Autodesk Inventor part; units mm, degrees
ref_plane "작업 평면1" through (80, 0, 4.95) normal (0, 0, 1) x (1, 0, 0)
ref_plane "YZ Plane" through (0, 0, 0) normal (1, 0, 0) x (0, 1, 0)
ref_plane "XZ Plane" through (0, 0, 0) normal (0, 1, 0) x (-1, 0, 0)
sketch "스케치1" plane through (0, 0, 0) normal (1, 0, 0) x (0, 1, 0)
  circle A0 centre (0, 0) radius 6
  dimension "d0" = 12
extrude "돌출1" add sketch "스케치1" along normal blind 80
sketch "스케치8" plane through (0, 0, 0) normal (-1, 0, 0) x (0, 0, 1)
  circle A0 centre (0, 0) radius 6
  circle A1 centre (0, 0) radius 4.95
  dimension "d26" = 9.9
extrude "돌출8" cut sketch "스케치8" against normal blind 18.6
sketch "스케치9" plane through (0, 0, 0) normal (-1, 0, 0) x (0, 0, 1)
  circle A0 centre (0, 0) radius 4.8
  circle A1 centre (0, 0) radius 4.95
  dimension "d29" = 9.6
extrude "돌출9" cut sketch "스케치9" against normal blind 9
sketch "스케치10" plane through (0, 0, 0) normal (-1, 0, 0) x (0, 0, 1)
  circle A0 centre (0, 0) radius 4.95
  circle A1 centre (0, 0) radius 4.8
  dimension "d32" = 9.9
extrude "돌출10" add sketch "스케치10" against normal blind 8
sketch "스케치11" plane through (80, 0, 0) normal (1, 0, 0) x (0, 0, -1)
  circle A0 centre (0, 0) radius 6
  circle A1 centre (0, 0) radius 4.95
  dimension "d35" = 9.9
extrude "돌출11" cut sketch "스케치11" against normal blind 26
sketch "스케치12" plane through (80, 0, 0) normal (1, 0, 0) x (0, 0, -1)
  circle A0 centre (0, 0) radius 4.95
  circle A1 centre (0, 0) radius 4.8
  dimension "d38" = 9.6
extrude "돌출12" cut sketch "스케치12" against normal blind 16.4
sketch "스케치13" plane through (80, 0, 0) normal (1, 0, 0) x (0, 0, -1)
  circle A0 centre (0, 0) radius 4.95
  circle A1 centre (0, 0) radius 4.8
  dimension "d41" = 9.9
extrude "돌출13" add sketch "스케치13" against normal blind 15.4
ref_plane "작업 평면1" through (80, 0, 4.95) normal (0, 0, 1) x (1, 0, 0)
sketch "스케치14" plane through (80, 0, 4.95) normal (0, 0, 1) x (1, 0, 0)
  line L0 (-1.3, -1.55) -> (-13.4, -1.55)
  line L1 (-13.4, -1.55) -> (-13.4, 1.55)
  line L2 (-13.4, 1.55) -> (-1.3, 1.55)
  line L3 (-1.3, 1.55) -> (-1.3, -1.55)
  line L4 (-15.4, 4.95) -> (-15.4, -4.95)
  line L5 (0, 4.95) -> (0, -4.95)
  line L6 (0, 0) -> (-15.4, 0)
  line L7 (-15.4, 4.8) -> (-15.4, -4.8)
  point P0 (-80, 0)
  dimension "d44" = 12.1
  dimension "d45" = 3.1
  dimension "d46" = 12.1
  dimension "d47" = 2
  dimension "d48" = 1.55
extrude "돌출14" cut sketch "스케치14" against normal blind 1.3
sketch "스케치15" plane through (54, 0, 0) normal (1, 0, 0) x (0, 0, -1)
  circle A0 centre (0, 0) radius 4.95
  circle A1 centre (0, 0) radius 6
  circle A2 centre (0, 0) radius 4.95
  circle A3 centre (0, 0) radius 4.95
  circle A4 centre (0, 0) radius 4.8
  dimension "d51" = 9.6
extrude "돌출15" cut sketch "스케치15" against normal blind 1 contours A0 | A1
sketch "스케치16" plane through (18.6, 0, 0) normal (-1, 0, 0) x (0, 0, 1)
  circle A0 centre (0, 0) radius 4.95
  circle A1 centre (0, 0) radius 6
  circle A2 centre (0, 0) radius 4.95
  circle A3 centre (0, 0) radius 4.8
  dimension "d54" = 9.6
extrude "돌출16" cut sketch "스케치16" against normal blind 1.1 contours A0 | A1
sketch "스케치17" plane through (19.7, 0, 0) normal (-1, 0, 0) x (0, 0, 1)
  circle A0 centre (0, 0) radius 4.8
  circle A1 centre (0, 0) radius 6
  circle A2 centre (0, 0) radius 4.95
  circle A3 centre (0, 0) radius 4.95
extrude "돌출17" cut sketch "스케치17" against normal blind 33.35 contours A1
properties part number "10PI축" material "철, 주조"
Model file for the job. Use its own axes, mm. A direction names the side the tool comes from. Give positions to 0.01 mm unless a question says otherwise; leave off trailing zeros. Write each loop counter-clockwise with the first axis right and the second up, starting at its lowest first coordinate (ties: lowest second). Pieces come first, ordered by that corner, then holes. Notation, with made-up numbers: M -15.75,-11 L -3.75,-11 A13 cw -3.75,8 Z; hole C 88.25,-1 d4. An arc over 180 degrees is marked long. One line per item, written item: value. Start each with the question number.
Q1. Drop flat-ended pins along their axis: pin 1 Ø0.8 at (x, z) = (71.5, 4.5) entering from +Y; pin 2 Ø3 at (x, y) = (46, 2) entering from -Z; pin 3 Ø0.5 at (x, z) = (72.5, 4) entering from -Y. Give the stop position or say it passes through.
Q2. Probe probe 1 along X at (y, z) = (4, -2.75); probe 2 along X at (y, z) = (0, 4); probe 3 along Y at (x, z) = (31, -1.25). List the from-to ranges inside material, lowest first. Write a range as [from, to].
Q3. Saw through at A-A, the plane x = 56. Write the cut outline in (y, z), plus the area to 3 significant figures.
Q4. 3-axis set-ups, long thin cutter, end or side, ignore diameter. For faces 4 (the cylindrical face through (53.51, 4.05, -2.58)), 5 (the flat face through (66.6, 0, 4)), 6 (the cylindrical face through (58.87, 1.49, -4.72)): which of +Z, -Z, +X, -X, +Y, -Y reach the whole face in a straight line?
Q5. Two-plate mould, pull along Y, no slides. Class faces 1 (the flat face through (78.7, 0, 4)), 2 (the cylindrical face through (64.11, 4.05, -2.58)), 3 (the flat face through (0, 0, 0)): +Y half, -Y half, draft (parallel to the pull), parting line (faces both ways), or undercut.
Output values:
1. pin 1: stops at y = 2.77
1. pin 2: stops at z = -4.92
1. pin 3: stops at y = -3.23
2. probe 1: x = [0, 8], [9, 18.6], [19.7, 53], [54, 63.6], [64.6, 80]
2. probe 2: x = [0, 66.6], [78.7, 80]
2. probe 3: y = [-4.79, 4.79]
3. outline: C 0,0 d9.9
3. area: 77.0 mm²
4. face 4: none
4. face 5: +Z
4. face 6: +X, -X
5. face 1: undercut
5. face 2: parting line
5. face 3: draft
